Autodesk Inventor part; units mm, degrees
ref_plane "YZ Plane" through (0, 0, 0) normal (1, 0, 0) x (0, 1, 0)
ref_plane "XZ Plane" through (0, 0, 0) normal (0, 1, 0) x (-1, 0, 0)
ref_plane "XY Plane" through (0, 0, 0) normal (0, 0, 1) x (1, 0, 0)
sketch "Sketch1" plane through (0, 0, 0) normal (0, 0, 1) x (1, 0, 0)
  circle A0 centre (-218.543, 11.2583) radius 1.841
  circle A1 centre (-155.8206, -2.8835) radius 1.841
  line L0 (-230.2092, -86.3504) -> (-227.6561, -85.8234)
  arc A2 (-218.6185, -8.9067) -> (-227.6561, -85.8234) centre (166.9594, -93.2007) ccw
  arc A3 (-205.5726, 0.7003) -> (-218.6185, -8.9067) centre (-206.6279, -11.5281) ccw
  arc A4 (-205.5726, 0.7003) -> (-161.7862, -4.929) centre (-174.5768, 68.6888) ccw
  arc A5 (-161.7862, -4.929) -> (-153.1858, -5.8609) centre (-156.6626, 2.2036) ccw
  arc A6 (-153.1858, -5.8609) -> (-153.782, 0.6635) centre (-154.5502, -2.6961) ccw
  arc A7 (-153.782, 0.6635) -> (-160.6438, -0.507) centre (-155.9827, -7.1338) ccw
  arc A8 (-214.3232, 20.5519) -> (-160.6438, -0.507) centre (-140.3024, 130.2877) ccw
  arc A9 (-214.3232, 20.5519) -> (-227.6561, 16.6026) centre (-219.3619, 13.0819) ccw
  arc A10 (-227.6561, 16.6026) -> (-227.6561, -100.5779) centre (-89.6281, -41.9876) ccw
  line L1 (-227.6561, -100.5779) -> (-230.2092, -86.3504)
  point P0 (0, 0)
  point P1 (-190.934, -110.2879)
extrude "Extrusion1" add sketch "Sketch1" along normal blind 14
sketch "Sketch2" plane through (0, 0, 14) normal (0, 0, 1) x (1, 0, 0)
  arc A0 (-226.9928, 4.3779) -> (-231.786, -82.917) centre (-90.6456, -46.8878) ccw
  arc A1 (-221.1828, 0) -> (-231.786, -82.917) centre (55.5969, -77.5303) ccw
  line L0 (-226.9928, 4.3779) -> (-221.1828, 0)
  arc A2 (-208.6913, 11.3499) -> (-164.5355, -2.5941) centre (-156.1757, 100.764) ccw
  arc A3 (-208.6913, 6.3406) -> (-164.5355, -2.5941) centre (-170.8567, 79.7445) ccw
  line L1 (-208.6913, 11.3499) -> (-208.6913, 6.3406)
  point P0 (0, 0)
extrude "Extrusion2" cut sketch "Sketch2" against normal blind 14
properties part number "Claw"
Can you work these out from the model? Positions are in its coordinate system, mm. A direction names the side the tool comes from. Coordinates: 2 decimals unless noted, no trailing zeros. Loops run counter-clockwise (first coordinate to the right, second up) from the corner with the lowest first, then second, coordinate; pieces in that order, holes last.
Item 1: Suppose I cut it at D-D (x = -210.5). Please give me the cut outline in (y, z), then the cut area to 3 significant figures.
Answers below:
outline: (0.12, 0) - (18.07, 0) - (18.07, 14) - (0.12, 14) - close
area: 251 mm2
Item 2: Please list where these lines run through material, in increasing order: L1, parallel to X at y = -8, z = 5.5; L2, parallel to X at y = -71.5, z = 4.5; L3, parallel to Y at x = -194, z = 12.75.
Answers below:
L1: x = -235.67 to -231.03, -223.3 to -218.38
L2: x = -236.64 to -234.22, -231.77 to -227.13
L3: y = -3.46 to 0.47, 4.21 to 9.3
Item 3: Suppose I cut it at A-A (x = -224). Please give me the cut outline in (y, z).
Answers below:
outline: (-39.1, 0) - (-10.87, 0) - (-10.87, 14) - (-39.1, 14) - close; (2.12, 0) - (20.81, 0) - (20.81, 14) - (2.12, 14) - close
Item 4: Suppose I cut it at C-C (z = 5). Please give me the cut outline in (x, y), then the cut area to 3 significant figures.
Answers below:
outline: (-230.21, -86.35) - (-227.66, -85.82) arc R394.69 cw to (-218.62, -8.91) arc R12.27 cw to (-205.57, 0.7) arc R74.72 ccw to (-161.79, -4.93) arc R8.78 ccw to (-153.19, -5.86) arc R3.45 ccw to (-153.78, 0.66) arc R8.1 ccw to (-160.64, -0.51) arc R132.37 cw to (-214.32, 20.55) arc R9.01 ccw to (-227.66, 16.6) arc R149.95 ccw to (-227.66, -100.58) - close; hole (-231.79, -82.92) arc R287.43 cw to (-221.18, 0) - (-226.99, 4.38) arc R145.67 ccw to start; hole circle Ø3.68 at (-218.54, 11.26); hole (-208.69, 6.34) arc R82.58 ccw to (-164.54, -2.59) arc R103.7 cw to (-208.69, 11.35) - close; hole circle Ø3.68 at (-155.82, -2.88)
area: 1,590 mm2
Item 5: I'm going to push flat-ended pins straight in: pin 1 (12 mm diameter, centred on x = -160, y = -18, fed in from +Z); pin 2 (6 mm diameter, centred on x = -155.82, y = -2.88, fed in from +Z); pin 3 (3 mm diameter, centred on y = -55.5, z = 4, fed in from +X); pin 4 (3 mm diameter, centred on y = -53.5, z = 1.5, fed in from +X). Where does each tip first touch, or does it pass through?
Answers below:
pin 1: passes through
pin 2: stops at z = 14
pin 3: stops at x = -225.77
pin 4: stops at x = -225.57
Item 6: Which directions (+Z, -Z, +X, -X, +Y, -Y) give clear straight access to the entire face, cutting with the end or side of a thin tool? Please do faces 1 (the face through (-222, -16, 0)), 2 (the face through (-228.915, -93.564, 6.902)).
Answers below:
face 1: -Z, +X, -X, +Y, -Y
face 2: +Z, -Z, +X
Item 7: Suppose I cut it at B-B (y = -51.5). Please give me the cut outline in (x, z), then the cut area to 3 significant figures.
Answers below:
outline: (-239.27, 0) - (-236.24, 0) - (-236.24, 14) - (-239.27, 14) - close; (-230.66, 0) - (-225.52, 0) - (-225.52, 14) - (-230.66, 14) - close
area: 114 mm2
Item 8: If we mould it in two halves opening along X, with no side actions, what happens to faces 3 (the face through (-222.03, 21.69, 6.9)), 4 (the face through (-208.691, 9, 7)), 5 (the face through (-229, -86.1, 6.9)), 6 (the face through (-224.1, 2.2, 7.1))? For each: released by +X, released by -X, zero draft, split by the parting line, or undercut.
Answers below:
face 3: split by the parting line
face 4: undercut
face 5: released by +X
face 6: undercut
